Geometry check sheet. Reference: the model listing, model coordinates, mm. A direction names the side the tool comes from. Coordinates: 2 decimals unless noted, no trailing zeros. Write each loop counter-clockwise with the first axis right and the second up, starting at its lowest first coordinate (ties: lowest second). Pieces come first, ordered by that corner, then holes. Notation, with made-up numbers: (15, 69) -> (58, 69) arc R16 ccw to (58, 81) -> close; hole circle Ø2 at (-34.5, 33.5). An arc over 180 degrees is marked (long way). Answer in a Markdown table with one row per item. Add a question column.
1. Set-up check for faces 1 (the cylindrical face through (-5.9, -3.4, 0)), 2 (the flat face through (-1.27, -2.9, 8.4)), 3 (the flat face through (0, -5.9, 8.4)): record each of +Z, -Z, +X, -X, +Y, -Y from which the full face is reachable in a straight line by a thin tool's end or side.
2. Mould release check, pull along X, two halves, no side actions. Record for faces 4 (the flat face through (1.27, -2.9, 8.4)), 5 (the flat face through (0, -6.9, -2)), 6 (the cylindrical face through (-0.195, -3.402, 3.452)): pulls with the +X half, pulls with the -X half, needs draft (parallel to the pull), parting line crosses it, or undercut.
3. Cross-section at A-A on x = 0. Record the cut outline in (y, z), and give its area (3 significant figures).
4. Cross-section at D-D on x = 5. Record the cut outline in (y, z) (3 decimals), and give its area (3 significant figures).
5. Cross-section at B-B on z = 0. Record the cut outline in (x, y), and give its area (3 significant figures).
6. Cross-section at C-C on z = -5. Record the cut outline in (x, y) (3 decimals), and give its area (3 significant figures).
7. Scan lines: L1, parallel to Z at x = 0, y = -4.5; L2, parallel to X at y = -5.75, z = 4; L3, parallel to X at y = -3.5, z = 4.25. Record each from-to range of solid material in increasing order. Write a range as from..to.
8. Depth check by flat-ended pin: P1, Ø0.8, axis at y = -3.5, z = 8.5, coming from the -X side; P2, Ø1.1, axis at x = 0.5, y = -6.5, coming from the +Z side; P3, Ø1.5, axis at y = -6, z = -2.5, coming from the +X side. Enter the tip coordinate at first touch or a pass-through.
```python
from build123d import *

# Parameters (mm, degrees)
F0_R     = 0.9
F1_DEPTH = 6.9
F2_W     = 1
F2_H     = 1
F3_DEPTH = 2.54


with BuildPart() as f1:
    # F0 (on Front) → F1 (new body)
    with BuildSketch(Plane.XZ):
        with BuildLine():
            Line((-1.27, 8.89855), (-1.27, 7.89855))
            ThreePointArc((-1.27, 7.89855), (0, -8), (1.27, 7.89855))
            Line((1.27, 7.89855), (1.27, 8.89855))
            Line((1.27, 8.89855), (-1.27, 8.89855))
        make_face()
        with Locations((-2.5, -4.330127)):
            Circle(F0_R, mode=Mode.SUBTRACT)
        with Locations((-5, 0)):
            Circle(F0_R, mode=Mode.SUBTRACT)
        with Locations((-3.75, -2.165064)):
            Circle(F0_R, mode=Mode.SUBTRACT)
        with Locations((-1.25, -2.165064)):
            Circle(F0_R, mode=Mode.SUBTRACT)
        with Locations((-2.5, 0)):
            Circle(F0_R, mode=Mode.SUBTRACT)
        with Locations((0, -4.330127)):
            Circle(F0_R, mode=Mode.SUBTRACT)
        with Locations((2.5, -4.330127)):
            Circle(F0_R, mode=Mode.SUBTRACT)
        with Locations((1.25, -2.165064)):
            Circle(F0_R, mode=Mode.SUBTRACT)
        with Locations((3.75, -2.165064)):
            Circle(F0_R, mode=Mode.SUBTRACT)
        Circle(F0_R, mode=Mode.SUBTRACT)
        with Locations((2.5, 0)):
            Circle(F0_R, mode=Mode.SUBTRACT)
        with Locations((5, 0)):
            Circle(F0_R, mode=Mode.SUBTRACT)
        with Locations((-3.75, 2.165064)):
            Circle(F0_R, mode=Mode.SUBTRACT)
        with Locations((-1.25, 2.165064)):
            Circle(F0_R, mode=Mode.SUBTRACT)
        with Locations((-2.5, 4.330127)):
            Circle(F0_R, mode=Mode.SUBTRACT)
        with Locations((1.25, 2.165064)):
            Circle(F0_R, mode=Mode.SUBTRACT)
        with Locations((3.75, 2.165064)):
            Circle(F0_R, mode=Mode.SUBTRACT)
        with Locations((0, 4.330127)):
            Circle(F0_R, mode=Mode.SUBTRACT)
        with Locations((2.5, 4.330127)):
            Circle(F0_R, mode=Mode.SUBTRACT)
    extrude(amount=F1_DEPTH)

    # F2 (on face) → F3 (cut)
    with BuildSketch(Plane(origin=(-1.27, 0, 0), x_dir=(0, -1, 0), z_dir=(-1, 0, 0))):
        with Locations((6.4, 8.39855)):
            Rectangle(F2_W, F2_H)
    extrude(amount=-F3_DEPTH, mode=Mode.SUBTRACT)


solid = f1.part
```
Results found:
| question | item | result |
|---|---|---|
| 1 | face 1 | +Y, -Y |
| 1 | face 2 | +Z, -X, +Y, -Y |
| 1 | face 3 | +Z, +X, -X, -Y |
| 2 | face 4 | pulls with the +X half |
| 2 | face 5 | needs draft |
| 2 | face 6 | undercut |
| 3 | outline | (-6.9, -8) -> (0, -8) -> (0, -5.23) -> (-6.9, -5.23) -> close; (-6.9, -3.43) -> (0, -3.43) -> (0, -0.9) -> (-6.9, -0.9) -> close; (-6.9, 0.9) -> (0, 0.9) -> (0, 3.43) -> (-6.9, 3.43) -> close; (-6.9, 5.23) -> (0, 5.23) -> (0, 8.9) -> (-5.9, 8.9) -> (-5.9, 7.9) -> (-6.9, 7.9) -> close |
| 3 | area | 78.3 mm^2 |
| 4 | outline | (-6.9, -6.245) -> (0, -6.245) -> (0, -0.9) -> (-6.9, -0.9) -> close; (-6.9, 0.9) -> (0, 0.9) -> (0, 6.245) -> (-6.9, 6.245) -> close |
| 4 | area | 73.8 mm^2 |
| 5 | outline | (-8, -6.9) -> (-5.9, -6.9) -> (-5.9, 0) -> (-8, 0) -> close; (-4.1, -6.9) -> (-3.4, -6.9) -> (-3.4, 0) -> (-4.1, 0) -> close; (-1.6, -6.9) -> (-0.9, -6.9) -> (-0.9, 0) -> (-1.6, 0) -> close; (0.9, -6.9) -> (1.6, -6.9) -> (1.6, 0) -> (0.9, 0) -> close; (3.4, -6.9) -> (4.1, -6.9) -> (4.1, 0) -> (3.4, 0) -> close; (5.9, -6.9) -> (8, -6.9) -> (8, 0) -> (5.9, 0) -> close |
| 5 | area | 48.3 mm^2 |
| 6 | outline | (-6.245, -6.9) -> (-3.101, -6.9) -> (-3.101, 0) -> (-6.245, 0) -> close; (-1.899, -6.9) -> (-0.601, -6.9) -> (-0.601, 0) -> (-1.899, 0) -> close; (0.601, -6.9) -> (1.899, -6.9) -> (1.899, 0) -> (0.601, 0) -> close; (3.101, -6.9) -> (6.245, -6.9) -> (6.245, 0) -> (3.101, 0) -> close |
| 6 | area | 61.3 mm^2 |
| 7 | L1 | z = -8..-5.23, -3.43..-0.9, 0.9..3.43, 5.23..8.9 |
| 7 | L2 | x = -6.93..-3.34, -1.66..-0.84, 0.84..1.66, 3.34..6.93 |
| 7 | L3 | x = -6.78..-3.4, -1.6..-0.9, 0.9..1.6, 3.4..6.78 |
| 8 | P1 | stops at x = -1.27 |
| 8 | P2 | stops at z = 7.9 |
| 8 | P3 | stops at x = 7.81 |
